```python
from build123d import *

# Parameters (mm, degrees)
SKIZZE1_W                        = 130
SKIZZE1_H                        = 180
AUFSATZ_LINEAR_AUSTRAGEN1_DEPTH  = 7
SKIZZE2_R                        = 20.5
SKIZZE2_R_2                      = 6
SKIZZE2_R_3                      = 2
AUFSATZ_LINEAR_AUSTRAGEN3_DEPTH  = 6
SKIZZE14_R                       = 20.5
SKIZZE14_R_2                     = 18.5
AUFSATZ_LINEAR_AUSTRAGEN14_DEPTH = 10
AUFSATZ_LINEAR_AUSTRAGEN4_DEPTH  = 59
SCHNITT_LINEAR_START             = 59
SKIZZE10_R                       = 18.5
SCHNITT_LINEAR_AUSTRAGEN3_DEPTH  = 59
SKIZZE11_R                       = 2
SKIZZE11_R_2                     = 6
SCHNITT_LINEAR_AUSTRAGEN4_DEPTH  = 6
SPIEGELN2_COPY_1_SKETCH_R        = 20.5
SPIEGELN2_COPY_1_SKETCH_R_2      = 6
SPIEGELN2_COPY_1_SKETCH_R_3      = 2
SPIEGELN2_COPY_1_DEPTH           = 6
SPIEGELN2_COPY_2_SKETCH_R        = 20.5
SPIEGELN2_COPY_2_SKETCH_R_2      = 18.5
SPIEGELN2_COPY_2_DEPTH           = 10
SPIEGELN2_COPY_3_DEPTH           = 59
SPIEGELN2_START                  = 59
SPIEGELN2_COPY_4_SKETCH_R        = 18.5
SPIEGELN2_COPY_4_DEPTH           = 59
SPIEGELN2_COPY_5_SKETCH_R        = 2
SPIEGELN2_COPY_5_SKETCH_R_2      = 6
SPIEGELN2_COPY_5_DEPTH           = 6
SPIEGELN2_COPY_6_SKETCH_R        = 20.5
SPIEGELN2_COPY_6_SKETCH_R_2      = 18.5
SPIEGELN2_COPY_6_DEPTH           = 10
SKIZZE13_R                       = 2
SCHNITT_LINEAR_AUSTRAGEN6_DEPTH  = 20
VERRUNDUNG1_R                    = 10


with BuildPart() as part:
    # Skizze1 → Aufsatz-Linear austragen1 (new body)
    with BuildSketch(Plane.XY):
        with Locations((65, 90)):
            Rectangle(SKIZZE1_W, SKIZZE1_H)
    extrude(amount=AUFSATZ_LINEAR_AUSTRAGEN1_DEPTH)

    # Skizze2 → Aufsatz-Linear austragen3 (add)
    with BuildSketch(Plane.ZY):
        with Locations((7, 140)):
            Circle(SKIZZE2_R)
        with Locations((0, 140)):
            Circle(SKIZZE2_R_2, mode=Mode.SUBTRACT)
        with Locations(Location((19.990381057, 147.5, 0), (0, 0, 270))):
            Circle(SKIZZE2_R_3, mode=Mode.SUBTRACT)
        with Locations(Location((19.990381057, 132.5, 0), (0, 0, 270))):
            Circle(SKIZZE2_R_3, mode=Mode.SUBTRACT)
        with Locations((7, 125)):
            Circle(SKIZZE2_R_3, mode=Mode.SUBTRACT)
        with Locations((7, 155)):
            Circle(SKIZZE2_R_3, mode=Mode.SUBTRACT)
        with Locations(Location((-5.990381057, 147.5, 0), (0, 0, 270))):
            Circle(SKIZZE2_R_3, mode=Mode.SUBTRACT)
        with Locations(Location((-5.990381057, 132.5, 0), (0, 0, 270))):
            Circle(SKIZZE2_R_3, mode=Mode.SUBTRACT)
    aufsatz_linear_austragen3 = extrude(amount=-AUFSATZ_LINEAR_AUSTRAGEN3_DEPTH)

    # Skizze14 → Aufsatz-Linear austragen14 (add)
    with BuildSketch(Plane(origin=(6, 0, 0), x_dir=(0, 0, -1), z_dir=(1, 0, 0))):
        with Locations((-7, 140)):
            Circle(SKIZZE14_R)
        with Locations((-7, 140)):
            Circle(SKIZZE14_R_2, mode=Mode.SUBTRACT)
    aufsatz_linear_austragen14 = extrude(amount=AUFSATZ_LINEAR_AUSTRAGEN14_DEPTH)

    # Skizze7 → Aufsatz-Linear austragen4 (add)
    with BuildSketch(Plane(origin=(6, 0, 0), x_dir=(0, 0, -1), z_dir=(1, 0, 0))):
        with BuildLine():
            Line((0, 159.267848868), (0, 157.12454379))
            ThreePointArc((0, 157.12454379), (-25.5, 140), (0, 122.87545621))
            Line((0, 122.87545621), (0, 120.732151132))
            ThreePointArc((0, 120.732151132), (-27.5, 140), (0, 159.267848868))
        make_face()
    aufsatz_linear_austragen4 = extrude(amount=AUFSATZ_LINEAR_AUSTRAGEN4_DEPTH)

    # Skizze10 → Schnitt-Linear austragen3 (cut)
    with BuildSketch(Plane.ZY.offset(-65).offset(SCHNITT_LINEAR_START)):
        with Locations(Location((7, 140, 0), (0, 0, 90))):
            Circle(SKIZZE10_R)
    schnitt_linear_austragen3 = extrude(amount=-SCHNITT_LINEAR_AUSTRAGEN3_DEPTH, mode=Mode.SUBTRACT)

    # Skizze11 → Schnitt-Linear austragen4 (cut)
    with BuildSketch(Plane.ZY):
        with Locations(Location((7, 155, 0), (0, 0, 270))):
            Circle(SKIZZE11_R)
        with Locations(Location((7, 125, 0), (0, 0, 270))):
            Circle(SKIZZE11_R)
        with Locations(Location((0, 140, 0), (0, 0, 270))):
            Circle(SKIZZE11_R_2)
    schnitt_linear_austragen4 = extrude(amount=-SCHNITT_LINEAR_AUSTRAGEN4_DEPTH, mode=Mode.SUBTRACT)

    # Spiegeln1: Aufsatz-Linear austragen3, Aufsatz-Linear austragen14, Aufsatz-Linear austragen4, Schnitt-Linear austragen3, Schnitt-Linear austragen4 across plane
    add(aufsatz_linear_austragen3.mirror(Plane.ZY.offset(-65)))
    add(aufsatz_linear_austragen14.mirror(Plane.ZY.offset(-65)))
    add(aufsatz_linear_austragen4.mirror(Plane.ZY.offset(-65)))
    add(schnitt_linear_austragen3.mirror(Plane.ZY.offset(-65)), mode=Mode.SUBTRACT)
    add(schnitt_linear_austragen4.mirror(Plane.ZY.offset(-65)), mode=Mode.SUBTRACT)

    # Spiegeln2: Aufsatz-Linear austragen3, Aufsatz-Linear austragen4, Schnitt-Linear austragen3, Schnitt-Linear austragen4 across plane
    add(aufsatz_linear_austragen3.mirror(Plane(origin=(0, 90, 0), x_dir=(0, 0, 1), z_dir=(0, -1, 0))))
    add(aufsatz_linear_austragen4.mirror(Plane(origin=(0, 90, 0), x_dir=(0, 0, 1), z_dir=(0, -1, 0))))
    add(schnitt_linear_austragen3.mirror(Plane(origin=(0, 90, 0), x_dir=(0, 0, 1), z_dir=(0, -1, 0))), mode=Mode.SUBTRACT)
    add(schnitt_linear_austragen4.mirror(Plane(origin=(0, 90, 0), x_dir=(0, 0, 1), z_dir=(0, -1, 0))), mode=Mode.SUBTRACT)

    # Spiegeln2 copy 1 sketch → Spiegeln2 copy 1 (add)
    with BuildSketch(Plane(origin=(130, 180, 0), x_dir=(0, 0, 1), z_dir=(1, 0, 0))):
        with Locations((7, 140)):
            Circle(SPIEGELN2_COPY_1_SKETCH_R)
        with Locations((0, 140)):
            Circle(SPIEGELN2_COPY_1_SKETCH_R_2, mode=Mode.SUBTRACT)
        with Locations(Location((19.990381057, 147.5, 0), (0, 0, 270))):
            Circle(SPIEGELN2_COPY_1_SKETCH_R_3, mode=Mode.SUBTRACT)
        with Locations(Location((19.990381057, 132.5, 0), (0, 0, 270))):
            Circle(SPIEGELN2_COPY_1_SKETCH_R_3, mode=Mode.SUBTRACT)
        with Locations((7, 125)):
            Circle(SPIEGELN2_COPY_1_SKETCH_R_3, mode=Mode.SUBTRACT)
        with Locations((7, 155)):
            Circle(SPIEGELN2_COPY_1_SKETCH_R_3, mode=Mode.SUBTRACT)
        with Locations(Location((-5.990381057, 147.5, 0), (0, 0, 270))):
            Circle(SPIEGELN2_COPY_1_SKETCH_R_3, mode=Mode.SUBTRACT)
        with Locations(Location((-5.990381057, 132.5, 0), (0, 0, 270))):
            Circle(SPIEGELN2_COPY_1_SKETCH_R_3, mode=Mode.SUBTRACT)
    extrude(amount=-SPIEGELN2_COPY_1_DEPTH)

    # Spiegeln2 copy 2 sketch → Spiegeln2 copy 2 (add)
    with BuildSketch(Plane(origin=(124, 180, 0), x_dir=(0, 0, -1), z_dir=(-1, 0, 0))):
        with Locations((-7, 140)):
            Circle(SPIEGELN2_COPY_2_SKETCH_R)
        with Locations((-7, 140)):
            Circle(SPIEGELN2_COPY_2_SKETCH_R_2, mode=Mode.SUBTRACT)
    extrude(amount=SPIEGELN2_COPY_2_DEPTH)

    # Spiegeln2 copy 3 sketch → Spiegeln2 copy 3 (add)
    with BuildSketch(Plane(origin=(124, 180, 0), x_dir=(0, 0, -1), z_dir=(-1, 0, 0))):
        with BuildLine():
            Line((0, 159.267848868), (0, 157.12454379))
            ThreePointArc((0, 157.12454379), (-25.5, 140), (0, 122.87545621))
            Line((0, 122.87545621), (0, 120.732151132))
            ThreePointArc((0, 120.732151132), (-27.5, 140), (0, 159.267848868))
        make_face()
    extrude(amount=SPIEGELN2_COPY_3_DEPTH)

    # Spiegeln2 copy 4 sketch → Spiegeln2 copy 4 (cut)
    with BuildSketch(Plane(origin=(65, 180, 0), x_dir=(0, 0, 1), z_dir=(1, 0, 0)).offset(SPIEGELN2_START)):
        with Locations(Location((7, 140, 0), (0, 0, 90))):
            Circle(SPIEGELN2_COPY_4_SKETCH_R)
    extrude(amount=-SPIEGELN2_COPY_4_DEPTH, mode=Mode.SUBTRACT)

    # Spiegeln2 copy 5 sketch → Spiegeln2 copy 5 (cut)
    with BuildSketch(Plane(origin=(130, 180, 0), x_dir=(0, 0, 1), z_dir=(1, 0, 0))):
        with Locations(Location((7, 155, 0), (0, 0, 270))):
            Circle(SPIEGELN2_COPY_5_SKETCH_R)
        with Locations(Location((7, 125, 0), (0, 0, 270))):
            Circle(SPIEGELN2_COPY_5_SKETCH_R)
        with Locations(Location((0, 140, 0), (0, 0, 270))):
            Circle(SPIEGELN2_COPY_5_SKETCH_R_2)
    extrude(amount=-SPIEGELN2_COPY_5_DEPTH, mode=Mode.SUBTRACT)

    # Spiegeln2 copy 6 sketch → Spiegeln2 copy 6 (add)
    with BuildSketch(Plane(origin=(6, 180, 0), x_dir=(0, 0, -1), z_dir=(1, 0, 0))):
        with Locations((-7, -140)):
            Circle(SPIEGELN2_COPY_6_SKETCH_R)
        with Locations((-7, -140)):
            Circle(SPIEGELN2_COPY_6_SKETCH_R_2, mode=Mode.SUBTRACT)
    extrude(amount=SPIEGELN2_COPY_6_DEPTH)

    # Skizze13 → Schnitt-Linear austragen6 (cut)
    with BuildSketch(Plane(origin=(0, 0, 0), x_dir=(-1, 0, 0), z_dir=(0, 0, -1))):
        with Locations((-12.5, 112.5)):
            Circle(SKIZZE13_R)
        with Locations((-27.5, 112.5)):
            Circle(SKIZZE13_R)
        with Locations((-42.5, 112.5)):
            Circle(SKIZZE13_R)
        with Locations((-57.5, 112.5)):
            Circle(SKIZZE13_R)
        with Locations((-72.5, 112.5)):
            Circle(SKIZZE13_R)
        with Locations((-87.5, 112.5)):
            Circle(SKIZZE13_R)
        with Locations((-102.5, 112.5)):
            Circle(SKIZZE13_R)
        with Locations((-117.5, 112.5)):
            Circle(SKIZZE13_R)
        with Locations((-27.5, 97.5)):
            Circle(SKIZZE13_R)
        with Locations((-42.5, 97.5)):
            Circle(SKIZZE13_R)
        with Locations((-57.5, 97.5)):
            Circle(SKIZZE13_R)
        with Locations((-72.5, 97.5)):
            Circle(SKIZZE13_R)
        with Locations((-87.5, 97.5)):
            Circle(SKIZZE13_R)
        with Locations((-102.5, 97.5)):
            Circle(SKIZZE13_R)
        with Locations((-117.5, 97.5)):
            Circle(SKIZZE13_R)
        with Locations((-27.5, 82.5)):
            Circle(SKIZZE13_R)
        with Locations((-42.5, 82.5)):
            Circle(SKIZZE13_R)
        with Locations((-57.5, 82.5)):
            Circle(SKIZZE13_R)
        with Locations((-72.5, 82.5)):
            Circle(SKIZZE13_R)
        with Locations((-87.5, 82.5)):
            Circle(SKIZZE13_R)
        with Locations((-102.5, 82.5)):
            Circle(SKIZZE13_R)
        with Locations((-117.5, 82.5)):
            Circle(SKIZZE13_R)
        with Locations((-27.5, 67.5)):
            Circle(SKIZZE13_R)
        with Locations((-42.5, 67.5)):
            Circle(SKIZZE13_R)
        with Locations((-57.5, 67.5)):
            Circle(SKIZZE13_R)
        with Locations((-72.5, 67.5)):
            Circle(SKIZZE13_R)
        with Locations((-87.5, 67.5)):
            Circle(SKIZZE13_R)
        with Locations((-102.5, 67.5)):
            Circle(SKIZZE13_R)
        with Locations((-117.5, 67.5)):
            Circle(SKIZZE13_R)
        with Locations((-12.5, 97.5)):
            Circle(SKIZZE13_R)
        with Locations((-12.5, 82.5)):
            Circle(SKIZZE13_R)
        with Locations((-12.5, 67.5)):
            Circle(SKIZZE13_R)
        with Locations((-117.5, 169.633924434)):
            Circle(SKIZZE13_R)
        with Locations((-102.5, 169.633924434)):
            Circle(SKIZZE13_R)
        with Locations((-87.5, 169.633924434)):
            Circle(SKIZZE13_R)
        with Locations((-72.5, 169.633924434)):
            Circle(SKIZZE13_R)
        with Locations((-57.5, 169.633924434)):
            Circle(SKIZZE13_R)
        with Locations((-42.5, 169.633924434)):
            Circle(SKIZZE13_R)
        with Locations((-27.5, 169.633924434)):
            Circle(SKIZZE13_R)
        with Locations((-12.5, 169.633924434)):
            Circle(SKIZZE13_R)
        with Locations((-12.5, 10.366075566)):
            Circle(SKIZZE13_R)
        with Locations((-27.5, 10.366075566)):
            Circle(SKIZZE13_R)
        with Locations((-42.5, 10.366075566)):
            Circle(SKIZZE13_R)
        with Locations((-57.5, 10.366075566)):
            Circle(SKIZZE13_R)
        with Locations((-72.5, 10.366075566)):
            Circle(SKIZZE13_R)
        with Locations((-87.5, 10.366075566)):
            Circle(SKIZZE13_R)
        with Locations((-102.5, 10.366075566)):
            Circle(SKIZZE13_R)
        with Locations((-117.5, 10.366075566)):
            Circle(SKIZZE13_R)
    extrude(amount=-SCHNITT_LINEAR_AUSTRAGEN6_DEPTH, mode=Mode.SUBTRACT)

    # Verrundung1
    verrundung1_edges = [part.edges().sort_by_distance(p)[0] for p in [
        (0, 180, 3.5),
        (130, 180, 3.5),
        (130, 0, 3.5),
        (0, 0, 3.5),
    ]]
    fillet(verrundung1_edges, radius=VERRUNDUNG1_R)


solid = part.part
```
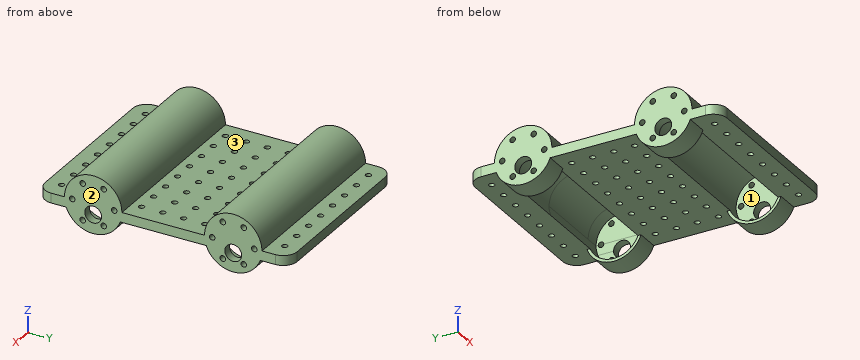
CAD build for the part. Positions are in the model's coordinates, mm. Face numbers are marked on the shaded views. Give positions to 0.01 mm unless a question says otherwise; leave off trailing zeros. Order: outer loops, then holes, each group sorted by start corner. A loop starts at its lowest first (then second) coordinate and runs counter-clockwise, first axis right, second up. Notation, with made-up numbers: M 89.25,-24.5 L 142.25,-24.5 A15 cw 142.25,-18.5 Z; hole C 39.5,-21.5 d5. An arc over 180 degrees is marked long. Put each result on its own line as item: value. Start each with the question number.
(1) Mould opens along X. For the marked faces 1, 2 and 3 say: +X half, -X half, draft (parallel to the pull), parting line (faces both ways), or undercut.
(2) Saw through at C-C, the plane x = 107. Write the cut outline in (y, z).
(3) Flat gauge pins, fed straight in: pin 1 Ø6 at (x, z) = (107, -5.5) entering from +Y; pin 2 Ø2 at (x, z) = (105.5, 19.5) entering from +Y; pin 3 Ø6.5 at (x, y) = (57.5, 97.5) entering from +Z; pin 4 Ø2 at (x, y) = (58, 72.5) entering from -Z. Where does each tip first touch, or does it go through?
(4) Saw through at B-B, the plane x = 72.5. Give the number of separate pieces and of enclosed holes in the cut face, then the cut area to 3 significant figures.
(5) Saw through at A-A, the plane y = 42. Write the cut outline in (x, z).
(6) Drill centre lines: line 1 along Y through (x, z) = (9, 14); line 2 along X through (y, z) = (153.5, 15); line 3 along Y through (x, z) = (110, 3). Where is each one in solid material? Low to high.
Check result:
1. face 1: undercut
1. face 2: +X half
1. face 3: draft
2. outline: M 0,0 L 22.88,0 A18.5 cw long 57.12,0 L 122.88,0 A18.5 cw long 157.12,0 L 180,0 L 180,7 L 160.5,7 A20.5 ccw 119.5,7 L 60.5,7 A20.5 ccw 19.5,7 L 0,7 Z
3. pin 1: passes through
3. pin 2: stops at y = 156.97
3. pin 3: stops at z = 7
3. pin 4: stops at z = 0
4. separate pieces: 7
4. enclosed holes: 0
4. area: 832 mm2
5. outline: M 0,-13.4 L 16,-13.4 L 16,-11.39 L 6,-11.39 L 6,-5.66 L 0,-5.66 Z; M 0,5.66 L 6,5.66 L 6,25.39 L 124,25.39 L 124,5.66 L 130,5.66 L 130,27.4 L 0,27.4 Z; M 114,-13.4 L 130,-13.4 L 130,-5.66 L 124,-5.66 L 124,-11.39 L 114,-11.39 Z
6. line 1: y = 20.73 to 22.88, 57.12 to 59.27, 120.73 to 122.88, 157.12 to 159.27
6. line 2: x = 0 to 6, 124 to 130
6. line 3: y = 0 to 21.94, 58.06 to 121.94, 158.06 to 180
